from build123d import *

# Parameters (mm, degrees)
CUT_EXTRUDE_1_DEPTH      = 19.987901745
CUT_EXTRUDE_1_DEPTH_BACK = 19.987901745
SKETCH_2_R               = 1.51
SKETCH_4_R               = 4.643686352
CUT_EXTRUDE_2_DEPTH      = 5
SKETCH_5_R               = 3.676903301
CUT_EXTRUDE_3_DEPTH      = 3
FILLET_1_R               = 1


with BuildPart() as part:
    # 草图1 → 旋转1 (revolve)
    with BuildSketch(Plane.XY):
        with BuildLine():
            Line((-1.222258531, -6.073377549), (-1.222258531, 7.441604752))
            Line((-1.222258531, 7.441604752), (-8.652530525, 7.441604752))
            ThreePointArc((-8.652530525, 7.441604752), (-8.933673585, -1.512962184), (-1.222258531, -6.073377549))
        make_face()
    revolve(axis=Axis((-1.222258531, 5.226622451, 0), (0, -1, 0)))

    # 草图2 → 切除-拉伸1 (cut, two sides: drawn at the far end of the back side and taken through both)
    with BuildSketch(Plane(origin=(0, 7.441604752, 0), x_dir=(1, 0, 0), z_dir=(0, 1, 0)).offset(-CUT_EXTRUDE_1_DEPTH_BACK)):
        with Locations(Location((-1.222258531, 0, 0), (0, 0, 270))):
            Circle(SKETCH_2_R)
    extrude(amount=CUT_EXTRUDE_1_DEPTH + CUT_EXTRUDE_1_DEPTH_BACK, mode=Mode.SUBTRACT)

    # 草图4 → 切除-拉伸2 (cut)
    with BuildSketch(Plane(origin=(0, -10, 0), x_dir=(1, 0, 0), z_dir=(0, 1, 0))):
        with Locations((-1.222258531, 0)):
            Circle(SKETCH_4_R)
    extrude(amount=CUT_EXTRUDE_2_DEPTH, mode=Mode.SUBTRACT)

    # 草图5 → 切除-拉伸3 (cut)
    with BuildSketch(Plane.XZ.offset(5)):
        with Locations(Location((-1.222258531, 0, 0), (0, 0, 270))):
            Circle(SKETCH_5_R)
    extrude(amount=-CUT_EXTRUDE_3_DEPTH, mode=Mode.SUBTRACT)

    # 圆角1
    fillet_1_edges = [part.edges().sort_by_distance(p)[0] for p in [
        (6.208013462, 7.441604752, 0),
    ]]
    fillet(fillet_1_edges, radius=FILLET_1_R)


solid = part.part
For this review, take the finished solid that the model builds, in its own axes (mm). A direction names the side the tool comes from. Round coordinates to 2 decimals unless told otherwise and drop trailing zeros. Order: outer loops, then holes, each group sorted by start corner. A loop starts at its lowest first (then second) coordinate and runs counter-clockwise, first axis right, second up. Notation, with made-up numbers: (23, -27.5) -> (35, -27.5) arc R20 ccw to (35, -13.5) -> close; hole circle Ø3 at (51.25, 68). An arc over 180 degrees is marked (long way). Put each result on its own line as item: value.
Q1. Add section B-B on y = -0.75. Write out the cut boundary in (x, z).
Check result:
outline: circle Ø16.17 at (-1.22, 0); hole circle Ø3.02 at (-1.22, 0)
Q2. Add section A-A on y = 1.5. Write out the cut boundary in (x, z), plus the area to 3 significant figures.
Check result:
outline: circle Ø17.43 at (-1.22, 0); hole circle Ø3.02 at (-1.22, 0)
area: 231 mm2
Q3. For probe 1 along Y at (x, z) = (-2, 1.75); probe 2 along X at (y, z) = (3.25, 0); probe 3 along Z at (x, y) = (0.75, -3), list the stretches that pass through material, from the lowest coordinate up. Write a range as [from, to].
Check result:
probe 1: [-2, 7.44]
probe 2: [-10.01, -2.73], [0.29, 7.56]
probe 3: [-6.38, -3.1], [3.1, 6.38]
Q4. Machinability: for faces 1 (the cylindrical face through (0.275, 2.655, -0.197)), 2 (the cylindrical face through (-4.81, -3.52, 0.8)), which of the approach directions +Z, -Z, +X, -X, +Y, -Y give a long, thin tool a straight path to every point of the face, cutting with its end or side? Answer none if there is none.
Check result:
face 1: +Y, -Y
face 2: -Y
Q5. Insertion check: pin 1 Ø1.5 at (x, y) = (2, 0.5) entering from -Z; pin 2 Ø3.5 at (x, z) = (-0.5, 0.5) entering from -Y; pin 3 Ø1 at (y, z) = (0, -7) entering from -X. Each pin has a flat end and moves straight along its axis. Give the tip position at first contact, or say it passes through.
Check result:
pin 1: z = -8.21
pin 2: y = -2
pin 3: x = -6.54
Q6. Mouldability with a two-part tool opening along X and no side actions: class faces 3 (the flat face through (-3, 7.442, 0)), 4 (the flat face through (-1, -2, -2)) as pulls with the +X half, pulls with the -X half, needs draft (parallel to the pull), parting line crosses it, or undercut.
Check result:
face 3: needs draft
face 4: undercut
